Read the model definition and answer for the solid it produces. Units are mm, in the model's axes. A direction names the side the tool comes from. Give positions to 0.01 mm unless a question says otherwise; leave off trailing zeros. Loops run counter-clockwise (first coordinate to the right, second up) from the corner with the lowest first, then second, coordinate; pieces in that order, holes last. Notation, with made-up numbers: (-36.5, 63.25) - (2.5, 63.25) arc R31 cw to (2.5, 95.25) - close; hole circle Ø8 at (87.5, -31). An arc over 180 degrees is marked (long way). Put each result on its own line as item: value. Start each with the question number.
1. For a pull along Z with two mould halves and no side action, classify faces 4 (the flat face through (0, -11.2, 65)), 5 (the cylindrical face through (23.497, 0.268, 125.93)), 6 (the flat face through (0, 11.2, 65)), 7 (the flat face through (0, 0, 132)) as released by +Z, released by -Z, zero draft, split by the parting line, or undercut.
2. Consider L1, parallel to Y at x = 10.5, z = 27; L2, parallel to X at y = 6.75, z = 112; L3, parallel to X at y = -7.75, z = 71.5. Determine where each line is inside the solid, lowest interval first. Write a range as from..to.
3. A cutting plane is placed at C-C, the plane z = 45. Determine the outline of the cut face in (x, y), plus the area to 3 significant figures.
4. For faces 1 (the cylindrical face through (22.5, 0.2, 65.2)), 2 (the cylindrical face through (-23.497, -0.268, 125.93)), 3 (the cylindrical face through (-22.5, -0.2, 65.2)), determine the directions among +Z, -Z, +X, -X, +Y, -Y from which every point of the face is accessible in a straight line to the end or side of a thin tool.
5. Given pin 1 Ø5 at (x, z) = (-15.5, 84) entering from -Y; pin 2 Ø1.5 at (y, z) = (9.5, 69) entering from -X; pin 3 Ø10 at (y, z) = (7.5, 72.5) entering from +X, each flat-ended and moving along its own axis, determine where each tip first touches the part or whether it passes through.
```python
from build123d import *

# Parameters (mm, degrees)
EXTRUDE_1_DEPTH     = 132
CUT_EXTRUDE_1_DEPTH = 108
FILLET_1_R          = 1


with BuildPart() as part:
    # 草图1 → 凸台-拉伸1 (new body)
    with BuildSketch(Plane.XY):
        with BuildLine():
            Line((-11.3, 12.2), (11.3, 12.2))
            ThreePointArc((11.3, 12.2), (23.5, 0), (11.3, -12.2))
            Line((11.3, -12.2), (-11.3, -12.2))
            ThreePointArc((-11.3, -12.2), (-23.5, 0), (-11.3, 12.2))
        make_face()
    extrude(amount=EXTRUDE_1_DEPTH)

    # 草图2 → 切除-拉伸1 (cut)
    with BuildSketch(Plane(origin=(0, 0, 12), x_dir=(-1, 0, 0), z_dir=(0, 0, -1))):
        with BuildLine():
            Line((11.3, 12.2), (-11.3, 12.2))
            ThreePointArc((-11.3, 12.2), (-23.5, 0), (-11.3, -12.2))
            Line((-11.3, -12.2), (11.3, -12.2))
            ThreePointArc((11.3, -12.2), (23.5, 0), (11.3, 12.2))
        make_face()
        with BuildLine():
            Line((11.3, 11.2), (-11.3, 11.2))
            ThreePointArc((-11.3, 11.2), (-22.5, 0), (-11.3, -11.2))
            Line((-11.3, -11.2), (11.3, -11.2))
            ThreePointArc((11.3, -11.2), (22.5, 0), (11.3, 11.2))
        make_face(mode=Mode.SUBTRACT)
    extrude(amount=-CUT_EXTRUDE_1_DEPTH, mode=Mode.SUBTRACT)

    # 圆角1
    fillet_1_edges = [part.edges().sort_by_distance(p)[0] for p in [
        (23.5, 0, 132),
        (0, 12.2, 132),
        (-23.5, 0, 120),
        (0, -12.2, 120),
        (23.5, 0, 120),
        (0, 12.2, 120),
        (-23.5, 0, 12),
        (0, 12.2, 12),
        (23.5, 0, 12),
        (0, -12.2, 12),
        (-23.5, 0, 132),
        (0, 12.2, 0),
        (23.5, 0, 0),
        (0, -12.2, 0),
        (-23.5, 0, 0),
        (0, -12.2, 132),
    ]]
    fillet(fillet_1_edges, radius=FILLET_1_R - 0.0001)  # a hair under: the kernel refuses the full size


solid = part.part
```
Return value:
1. face 4: undercut
1. face 5: zero draft
1. face 6: undercut
1. face 7: released by +Z
2. L1: y = -11.2..11.2
2. L2: x = -20.24..20.24
2. L3: x = -19.39..19.39
3. outline: (-11.3, -11.2) - (11.3, -11.2) arc R11.2 ccw to (11.3, 11.2) - (-11.3, 11.2) arc R11.2 ccw to start
3. area: 900 mm2
4. face 1: +X
4. face 2: +Z, -Z, -X
4. face 3: -X
5. pin 1: stops at y = -11.07
5. pin 2: stops at x = -18.29
5. pin 3: stops at x = 22.22
